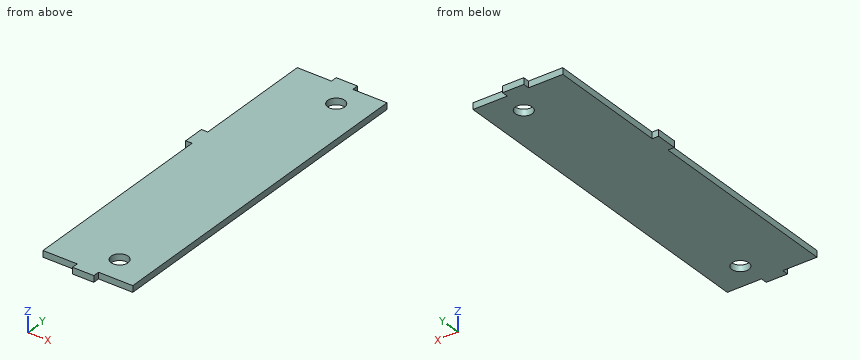
```python
from build123d import *

# Parameters (mm, degrees)
BOSS_EXTRUDE1_DEPTH      = 1.5
F_8_0_8_DIAMETER_HOLE1_D = 8


with BuildPart() as part:
    # Sketch1 → Boss-Extrude1 (new, symmetric)
    with BuildSketch(Plane.XY):
        Polygon((-5, 0), (5, 0), (5, -3), (21.1, -3), (21.1, -165), (5, -165), (5, -168), (-5, -168), (-5, -165), (-21.1, -165), (-21.1, -70), (-24.1, -70), (-24.1, -60), (-21.1, -60), (-21.1, -3), (-5, -3), align=None)
    extrude(amount=BOSS_EXTRUDE1_DEPTH, both=True)

    # Ø8.0 (8) Diameter Hole1 (through all)
    with Locations(Plane.XY.offset(1.5)):
        with Locations((6, -14.9), (6, -152.9)):
            Hole(F_8_0_8_DIAMETER_HOLE1_D / 2)


solid = part.part
```
Work out the finished part from the listing and answer in its coordinate system (mm). Round coordinates to 2 decimals unless told otherwise and drop trailing zeros. Write each loop counter-clockwise with the first axis right and the second up, starting at its lowest first coordinate (ties: lowest second). Pieces come first, ordered by that corner, then holes.
1) Flat-ended cylindrical pins translate along their axes: P1, Ø1.5, axis at y = -2, z = -0.5, coming from the +X side; P2, Ø0.9, axis at y = -33, z = 0, coming from the -X side; P3, Ø0.9, axis at x = 11.5, z = -0.5, coming from the -Y side. Find the tip coordinate at first contact, or state that the pin passes through.
2) A cutting plane is placed at B-B on z = -0.65. Determine the outline of the cut face in (x, y), and give its area (3 significant figures).
3) A cutting plane is placed at D-D on y = -141.5. Determine the outline of the cut face in (x, z), and give its area (3 significant figures).
4) Consider probe 1 along Y at (x, z) = (6, -0.45); probe 2 along X at (y, z) = (-78.5, -0.75); probe 3 along Y at (x, z) = (12, -1). Determine where each line is inside the solid, lowest interval first.
5) A cutting plane is placed at A-A on y = -14.9. Determine the outline of the cut face in (x, z), and give its area (3 significant figures).
6) A cutting plane is placed at C-C on x = -8.5. Determine the outline of the cut face in (y, z).
Entries:
1. P1: stops at x = 5
1. P2: stops at x = -21.1
1. P3: stops at y = -165
2. outline: (-24.1, -70) - (-21.1, -70) - (-21.1, -165) - (-5, -165) - (-5, -168) - (5, -168) - (5, -165) - (21.1, -165) - (21.1, -3) - (5, -3) - (5, 0) - (-5, 0) - (-5, -3) - (-21.1, -3) - (-21.1, -60) - (-24.1, -60) - close; hole circle Ø8 at (6, -152.9); hole circle Ø8 at (6, -14.9)
2. area: 6,830 mm2
3. outline: (-21.1, -1.5) - (21.1, -1.5) - (21.1, 1.5) - (-21.1, 1.5) - close
3. area: 127 mm2
4. probe 1: y = -165 to -156.9, -148.9 to -18.9, -10.9 to -3
4. probe 2: x = -21.1 to 21.1
4. probe 3: y = -165 to -3
5. outline: (-21.1, -1.5) - (2, -1.5) - (2, 1.5) - (-21.1, 1.5) - close; (10, -1.5) - (21.1, -1.5) - (21.1, 1.5) - (10, 1.5) - close
5. area: 103 mm2
6. outline: (-165, -1.5) - (-3, -1.5) - (-3, 1.5) - (-165, 1.5) - close
